CAD build for the part. Positions are in the model's coordinates, mm. A direction names the side the tool comes from. Round coordinates to 2 decimals unless told otherwise and drop trailing zeros. Write each loop counter-clockwise with the first axis right and the second up, starting at its lowest first coordinate (ties: lowest second). Pieces come first, ordered by that corner, then holes. Notation, with made-up numbers: (85, 41) - (99, 41) arc R23 cw to (99, 55) - close; hole circle Ø4 at (-8.75, -36.75). An arc over 180 degrees is marked (long way). Use one line per item in the form item = value. Start each with the question number.
Item 1: Drill centre lines: L1, parallel to Y at x = 0, z = 27.75; L2, parallel to X at y = 1.25, z = 2.5; L3, parallel to X at y = 0.5, z = 41. Where is each one in solid material? Low to high.
Item 2: Band-saw the part on B-B, the plane y = 2.5. List the corners of the cut face in (x, z), and give its area (3 significant figures).
Item 3: Band-saw the part on A-A, the plane z = 35. List the corners of the cut face in (x, y), and give its area (3 significant figures).
Item 4: Pin check, flat tips, straight feed: pin 1 (1 mm diameter, centred on y = 8, z = 24.5, fed in from -X); pin 2 (6 mm diameter, centred on x = 4.5, z = 22.5, fed in from +Y); pin 3 (1 mm diameter, centred on x = 2.5, z = 50.5, fed in from +Y). Stop position of each tip, or through.
Item 5: Pull direction Y, two halves, no side cores. Call faces 5 (the cylindrical face through (-7, 6.87, 3.32)), 6 (the flat face through (-5, 6, 4)), 7 (the cylindrical face through (7.847, 7.909, 26.328)): +Y half, -Y half, draft (parallel to the pull), parting line (faces both ways), or undercut.
Item 6: Tool access for faces 1 (the flat face through (-7, 10, 7.2)), 2 (the flat face through (6, -6, 51)), 3 (the cylindrical face through (0.206, -6.497, 6.592)), 4 (the flat face through (-6, -6, 51)): list every direction of +Z, -Z, +X, -X, +Y, -Y with a clear straight run to the whole face (end or side of a thin tool).
Item 7: Band-saw the part on C-C, the plane z = 3.6. Give the number of separate pieces and of enclosed holes in the cut face, and give its area (3 significant figures).
from build123d import *

# Parameters (mm, degrees)
BOSS_EXTRUDE1_DEPTH = 46
SKETCH3_R           = 6.5
BOSS_EXTRUDE2_DEPTH = 10
CUT_EXTRUDE7_DEPTH  = 6
CIRPATTERN1_COUNT   = 4
SKETCH12_R          = 6.5
CUT_EXTRUDE8_DEPTH  = 30
BOSS_EXTRUDE3_DEPTH = 7.2
SKETCH17_R          = 1.655
CUT_EXTRUDE10_DEPTH = 30
SKETCH18_R          = 5
CUT_EXTRUDE11_DEPTH = 6
BOSS_EXTRUDE4_DEPTH = 6
CIRPATTERN2_COUNT   = 36
SKETCH20_R          = 6.5
CUT_EXTRUDE12_DEPTH = 1.2
SKETCH21_W          = 10
SKETCH21_H          = 17.493725323
CUT_EXTRUDE13_DEPTH = 7.2


with BuildPart() as part:
    # Sketch1 → Boss-Extrude1 (new body)
    with BuildSketch(Plane.XY):
        with BuildLine():
            Line((-5.05, 9.05), (5.05, 9.05))
            ThreePointArc((5.05, 9.05), (7.878427125, 7.878427125), (9.05, 5.05))
            Line((9.05, 5.05), (9.05, -5.05))
            ThreePointArc((9.05, -5.05), (7.878427125, -7.878427125), (5.05, -9.05))
            Line((5.05, -9.05), (-5.05, -9.05))
            ThreePointArc((-5.05, -9.05), (-7.878427125, -7.878427125), (-9.05, -5.05))
            Line((-9.05, -5.05), (-9.05, 5.05))
            ThreePointArc((-9.05, 5.05), (-7.878427125, 7.878427125), (-5.05, 9.05))
        make_face()
    extrude(amount=BOSS_EXTRUDE1_DEPTH)

    # Sketch3 → Boss-Extrude2 (add)
    with BuildSketch(Plane.XY.offset(46)):
        Polygon((-5, -7), (5, -7), (7, -5), (7, 5), (5, 7), (-5, 7), (-7, 5), (-7, -5), align=None)
        Circle(SKETCH3_R, mode=Mode.SUBTRACT)
    extrude(amount=BOSS_EXTRUDE2_DEPTH)

    # Sketch11 → Cut-Extrude7 (cut)
    with BuildSketch(Plane.XY.offset(56)):
        Polygon((0, 0), (7, 0.45), (7, -0.45), align=None)
    cut_extrude7 = extrude(amount=-CUT_EXTRUDE7_DEPTH, mode=Mode.SUBTRACT)

    # CirPattern1: Cut-Extrude7 ×4 about axis
    cirpattern1_axis = Axis((0, 0, 56), (0, 0, -1))
    for i in range(1, CIRPATTERN1_COUNT):
        add(cut_extrude7.rotate(cirpattern1_axis, i * 360 / CIRPATTERN1_COUNT), mode=Mode.SUBTRACT)

    # Sketch12 → Cut-Extrude8 (cut)
    with BuildSketch(Plane.XY.offset(46)):
        with Locations((0, 0.192488852)):
            Circle(SKETCH12_R)
    extrude(amount=-CUT_EXTRUDE8_DEPTH, mode=Mode.SUBTRACT)

    # Sketch15 → Boss-Extrude3 (add)
    with BuildSketch(Plane.XY):
        with BuildLine():
            Line((-5.05, -9.05), (5.05, -9.05))
            ThreePointArc((5.05, -9.05), (7.878427125, -7.878427125), (9.05, -5.05))
            Line((9.05, -5.05), (9.05, 8))
            ThreePointArc((9.05, 8), (7.878427125, 10.828427125), (5.05, 12))
            Line((5.05, 12), (-5.05, 12))
            ThreePointArc((-5.05, 12), (-7.878427125, 10.828427125), (-9.05, 8))
            Line((-9.05, 8), (-9.05, -5.05))
            ThreePointArc((-9.05, -5.05), (-7.878427125, -7.878427125), (-5.05, -9.05))
        make_face()
    extrude(amount=BOSS_EXTRUDE3_DEPTH)

    # Sketch17 → Cut-Extrude10 (cut)
    with BuildSketch(Plane(origin=(9.05, 0, 0), x_dir=(0, 0, -1), z_dir=(1, 0, 0))):
        with Locations(Location((-3.6, 8.5, 0), (0, 0, 342.4153325))):
            Circle(SKETCH17_R)
    extrude(amount=-CUT_EXTRUDE10_DEPTH, mode=Mode.SUBTRACT)

    # Sketch18 → Cut-Extrude11 (cut)
    with BuildSketch(Plane.XY):
        Circle(SKETCH18_R)
    extrude(amount=CUT_EXTRUDE11_DEPTH, mode=Mode.SUBTRACT)

    # Sketch19 → Boss-Extrude4 (add)
    with BuildSketch(Plane.XY):
        with BuildLine():
            Line((-0.5, 4.974937186), (0, 4.455493066))
            Line((0, 4.455493066), (0.5, 4.974937186))
            ThreePointArc((0.5, 4.974937186), (0, 5.474937186), (-0.5, 4.974937186))
        make_face()
    boss_extrude4 = extrude(amount=BOSS_EXTRUDE4_DEPTH)

    # CirPattern2: Boss-Extrude4 ×36 about axis
    cirpattern2_axis = Axis((0, 0, 0), (0, 0, 1))
    for i in range(1, CIRPATTERN2_COUNT):
        add(boss_extrude4.rotate(cirpattern2_axis, i * 360 / CIRPATTERN2_COUNT))

    # Sketch20 → Cut-Extrude12 (cut)
    with BuildSketch(Plane(origin=(0, 0, 6), x_dir=(-1, 0, 0), z_dir=(0, 0, -1))):
        with Locations(Location((0, 0, 0), (0, 0, 0.848400141))):
            Circle(SKETCH20_R)
    extrude(amount=-CUT_EXTRUDE12_DEPTH, mode=Mode.SUBTRACT)

    # Sketch21 → Cut-Extrude13 (cut)
    with BuildSketch(Plane.XY):
        with Locations((0, 8.746862661)):
            Rectangle(SKETCH21_W, SKETCH21_H)
    extrude(amount=CUT_EXTRUDE13_DEPTH, mode=Mode.SUBTRACT)


solid = part.part
Determined:
q1.L1 = -9.05 to -6.31, 6.69 to 9.05
q1.L2 = -9.05 to -5, 5 to 9.05
q1.L3 = -9.05 to -6.49, 6.49 to 9.05
q2.outline = (-9.05, 0) - (-5, 0) - (-5, 6) - (-6, 6) - (-6, 7.2) - (6, 7.2) - (6, 6) - (5, 6) - (5, 0) - (9.05, 0) - (9.05, 46) - (7, 46) - (7, 56) - (6, 56) - (6, 46) - (6.08, 46) - (6.08, 16) - (-6.08, 16) - (-6.08, 46) - (-6, 46) - (-6, 56) - (-7, 56) - (-7, 46) - (-9.05, 46) - close
q2.area = 414 mm²
q3.outline = (-9.05, -5.05) arc R4 ccw to (-5.05, -9.05) - (5.05, -9.05) arc R4 ccw to (9.05, -5.05) - (9.05, 5.05) arc R4 ccw to (5.05, 9.05) - (-5.05, 9.05) arc R4 ccw to (-9.05, 5.05) - close; hole circle Ø13 at (0, 0.19)
q3.area = 181 mm²
q4.pin_1 = -8.21
q4.pin_2 = 9.05
q4.pin_3 = 7
q5.face_5 = undercut
q5.face_6 = draft
q5.face_7 = +Y half
q6.face_1 = +Z, -X, +Y
q6.face_2 = +Z, +X, -Y
q6.face_3 = none
q6.face_4 = +Z, -X, -Y
q7.separate_pieces = 3
q7.enclosed_holes = 0
q7.area = 187 mm²
